Could you check a few things on this model? Use its own coordinates, in mm. Face numbers are marked on the shaded views. Round coordinates to 2 decimals unless told otherwise and drop trailing zeros. Loops run counter-clockwise (first coordinate to the right, second up) from the corner with the lowest first, then second, coordinate; pieces in that order, holes last. Notation, with made-up numbers: (18.5, 68) -> (43.5, 68) arc R28 cw to (43.5, 87) -> close; hole circle Ø8 at (22.5, 56). An arc over 180 degrees is marked (long way). One line per item, written item: value.
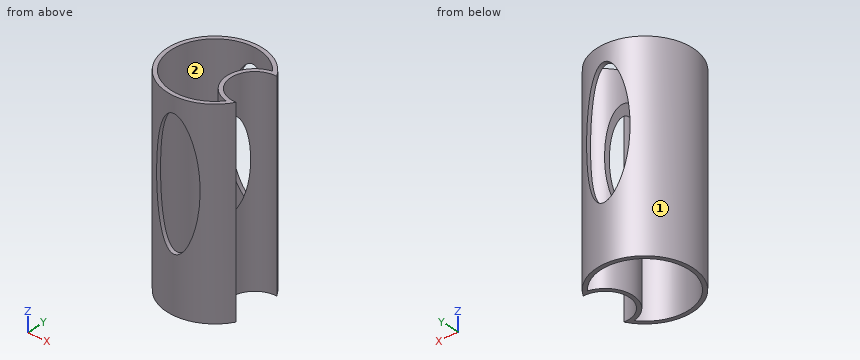
Autodesk Fusion 360 part; units mm, degrees
sketch "Sketch1" plane through (0, 0, 0) normal (0, 0, 1) x (1, 0, 0)
  circle A0 centre (0, 0) radius 6
  circle A1 centre (0, 0) radius 5.5
  circle A2 centre (4.9955, 0.0458) radius 3
  circle A3 centre (4.9955, 0.0458) radius 3.5
  dimension "d1" = 12
  dimension "d2" = 11
  dimension "d4" = 6
  dimension "d5" = 7
extrude "Extrude1" add sketch "Sketch1" along normal blind 25 contours A0 A1 A2 A3 | A0 A1 A2 A3 | A0 A1 A3 | A1 A2 A3
ref_plane "WorkPlane1" through (0, -6, 10.4032) normal (0, -1, 0) x (-1, 0, 0)
sketch "Sketch2" plane through (0, -6, 0) normal (0, -1, 0) x (-1, 0, 0)
  ellipse E0 centre (0, -15) end of major axis (0, -23) minor radius 2.75
  line L0 (0, -7) -> (0, -23) construction
  line L1 (-2.75, -15) -> (2.75, -15) construction
  dimension "d9" = 5.5
extrude "Extrude2" cut sketch "Sketch2" against normal blind 20
sketch "Sketch3" plane through (0, 0, 0) normal (0, 0, 1) x (1, 0, 0)
  line L0 (-63, 9) -> (-37, 9)
  line L1 (-37, 9) -> (-37, -12)
  line L2 (-37, -12) -> (-63, -12)
  line L3 (-63, -12) -> (-63, 9)
extrude "Extrude3" [suppressed]
sketch "Sketch4" plane through (0, -12, 0) normal (0, -1, 0) x (1, 0, 0)
  line L0 (-63, 0) -> (-37, 0)
  line L1 (-37, 0) -> (-37, 47)
  line L2 (-37, 47) -> (-63, 47)
  line L3 (-63, 47) -> (-63, 0)
  circle A0 centre (-54, 23) radius 2
  circle A1 centre (-54, 32) radius 2
  dimension "d14" = 4
  dimension "d15" = 4
  dimension "d16" = 9
  dimension "d17" = 15
  dimension "d18" = 23
equation "d2 = d1 - 1 mm"
(1) Thinking about a two-plate mould opening in X: for the marked faces 1 and 2, which applies, released by +X, released by -X, zero draft, split by the parting line, or undercut?
Recorded:
face 1: split by the parting line
face 2: undercut
(2) I'm going to push flat-ended pins straight in: pin 1 Ø5 at (y, z) = (4, 19.5) entering from +X; pin 2 Ø1.5 at (y, z) = (-5, 8.5) entering from -X; pin 3 Ø1.5 at (x, z) = (1, 6) entering from -Y; pin 4 Ø6.5 at (x, y) = (0, 0) entering from +Z. Where does each tip first touch, or does it pass through?
Recorded:
pin 1: x = 5.17
pin 2: x = -4.24
pin 3: y = -5.99
pin 4: z = 25
(3) If we section it at D-D, the plane z = 13: Give the number of separate pieces and of enclosed holes in the cut face, then the cut area to 3 significant figures.
Recorded:
separate pieces: 3
enclosed holes: 0
area: 11.5 mm²
(4) If we section it at B-B, the plane y = 4: Please give me the cut outline in (x, z), then the cut area to 3 significant figures.
Recorded:
outline: (-4.47, 0) -> (-3.77, 0) -> (-3.77, 25) -> (-4.47, 25) -> close; (3.77, 0) -> (4.47, 0) -> (4.47, 25) -> (3.77, 25) -> close
area: 34.9 mm²
(5) If we section it at A-A, the plane x = 3.5: Please give me the cut outline in (y, z).
Recorded:
outline: (-4.87, 0) -> (-4.24, 0) -> (-4.24, 25) -> (-4.87, 25) -> close; (-3.12, 0) -> (-2.55, 0) -> (-2.55, 25) -> (-3.12, 25) -> close; (2.65, 0) -> (3.21, 0) -> (3.21, 25) -> (2.65, 25) -> close; (4.24, 0) -> (4.87, 0) -> (4.87, 25) -> (4.24, 25) -> close
(6) If I drill on L1, parallel to Y at x = 4, z = 4.5; L2, parallel to Y at x = -2, z = 4; L3, parallel to Y at x = 3, z = 2.25, over which ranges is the centre line in solid material (lowest first)?
Recorded:
L1: -4.47 to -3.77, -3.31 to -2.78, 2.88 to 3.4, 3.77 to 4.47
L2: -5.66 to -5.12, 5.12 to 5.66
L3: -5.2 to -4.61, -2.83 to -2.19, 2.29 to 2.92, 4.61 to 5.2
